from build123d import *

# Parameters (mm, degrees)
BOSS_EXTRUDE1_DEPTH = 1.5
SKETCH2_R           = 3.1
CUT_EXTRUDE1_DEPTH  = 1.5


with BuildPart() as part:
    # Sketch1 → Boss-Extrude1 (new body)
    with BuildSketch(Plane(origin=(0, 0, 0), x_dir=(1, 0, 0), z_dir=(0, 1, 0))):
        with BuildLine():
            Line((2.414213562, 0), (69.385786438, 0))
            ThreePointArc((69.385786438, 0), (69.794034728, 0.211324865), (69.857190958, 0.666666667))
            ThreePointArc((69.857190958, 0.666666667), (70.092893219, 1.707106781), (71.133333333, 1.942809042))
            ThreePointArc((71.133333333, 1.942809042), (71.588675135, 2.005965272), (71.8, 2.414213562))
            Line((71.8, 2.414213562), (71.8, 34.385786438))
            ThreePointArc((71.8, 34.385786438), (71.588675135, 34.794034728), (71.133333333, 34.857190958))
            ThreePointArc((71.133333333, 34.857190958), (70.092893219, 35.092893219), (69.857190958, 36.133333333))
            ThreePointArc((69.857190958, 36.133333333), (69.794034728, 36.588675135), (69.385786438, 36.8))
            Line((69.385786438, 36.8), (2.414213562, 36.8))
            ThreePointArc((2.414213562, 36.8), (2.005965272, 36.588675135), (1.942809042, 36.133333333))
            ThreePointArc((1.942809042, 36.133333333), (1.707106781, 35.092893219), (0.666666667, 34.857190958))
            ThreePointArc((0.666666667, 34.857190958), (0.211324865, 34.794034728), (0, 34.385786438))
            Line((0, 34.385786438), (0, 2.414213562))
            ThreePointArc((0, 2.414213562), (0.211324865, 2.005965272), (0.666666667, 1.942809042))
            ThreePointArc((0.666666667, 1.942809042), (1.707106781, 1.707106781), (1.942809042, 0.666666667))
            ThreePointArc((1.942809042, 0.666666667), (2.005965272, 0.211324865), (2.414213562, 0))
        make_face()
    extrude(amount=BOSS_EXTRUDE1_DEPTH)

    # Sketch2 → Cut-Extrude1 (cut)
    with BuildSketch(Plane(origin=(0, 1.5, 0), x_dir=(1, 0, 0), z_dir=(0, 1, 0))):
        with Locations(Location((61.8, 7, 0), (0, 0, 270))):
            Circle(SKETCH2_R)
    extrude(amount=-CUT_EXTRUDE1_DEPTH, mode=Mode.SUBTRACT)


solid = part.part
Source: CAD feature listing. Evaluate the final solid. Frame: model axes, mm. Give positions to 0.01 mm unless a question says otherwise; leave off trailing zeros. Write each loop counter-clockwise with the first axis right and the second up, starting at its lowest first coordinate (ties: lowest second). Pieces come first, ordered by that corner, then holes. Notation, with made-up numbers: M 44,37.25 L 58,37.25 A21 cw 58,47.25 Z; hole C 67.5,74.5 d6. An arc over 180 degrees is marked long. Return JSON: item names as keys, results as strings. Group by question number.
1) Pin query (flat end, axial travel): P1, Ø3.5, axis at x = 61.8, z = -7, coming from the -Y side. Return the tip coordinate at first contact, or that it passes through.
2) Cut plane B-B, the plane x = 61.8. Output: boundary loops of the cut face in (y, z), plus the area to 3 significant figures.
3) Cut plane A-A, the plane z = -7. Output: boundary loops of the cut face in (x, y).
4) Material intervals for line 1 along X through (y, z) = (0.85, -7); line 2 along Z through (x, y) = (61.5, 0.9); line 3 along X through (y, z) = (0.35, -34.5), sorted ascending. Write a range as [from, to].
5) Pull-direction query (X, two-part tool) for faces 1 (the face through (35, 0, -19)), 2 (the face through (1.696, 0.74, -1.718)), 3 (the face through (0, 1, -19)), 4 (the face through (71.8, 1, -18)); classes: pulls with the +X half, pulls with the -X half, needs draft (parallel to the pull), parting line crosses it, or undercut.
6) Cut plane C-C, the plane y = 0.55. Output: boundary loops of the cut face in (x, z).
Recorded:
{
 "1": {"P1": "passes through"},
 "2": {"outline": "M 0,-36.8 L 1.5,-36.8 L 1.5,-10.1 L 0,-10.1 Z; M 0,-3.9 L 1.5,-3.9 L 1.5,0 L 0,0 Z", "area": "45.9 mm²"},
 "3": {"outline": "M 0,0 L 58.7,0 L 58.7,1.5 L 0,1.5 Z; M 64.9,0 L 71.8,0 L 71.8,1.5 L 64.9,1.5 Z"},
 "4": {"line 1": "x = [0, 58.7], [64.9, 71.8]", "line 2": "z = [-36.8, -10.09], [-3.91, 0]", "line 3": "x = [0.01, 71.79]"},
 "5": {"face 1": "needs draft", "face 2": "undercut", "face 3": "pulls with the -X half", "face 4": "pulls with the +X half"},
 "6": {"outline": "M 0,-34.39 A0.5 ccw 0.67,-34.86 A1 cw 1.94,-36.13 A0.5 ccw 2.41,-36.8 L 69.39,-36.8 A0.5 ccw 69.86,-36.13 A1 cw 71.13,-34.86 A0.5 ccw 71.8,-34.39 L 71.8,-2.41 A0.5 ccw 71.13,-1.94 A1 cw 69.86,-0.67 A0.5 ccw 69.39,0 L 2.41,0 A0.5 ccw 1.94,-0.67 A1 cw 0.67,-1.94 A0.5 ccw 0,-2.41 Z; hole C 61.8,-7 d6.2"}
}
